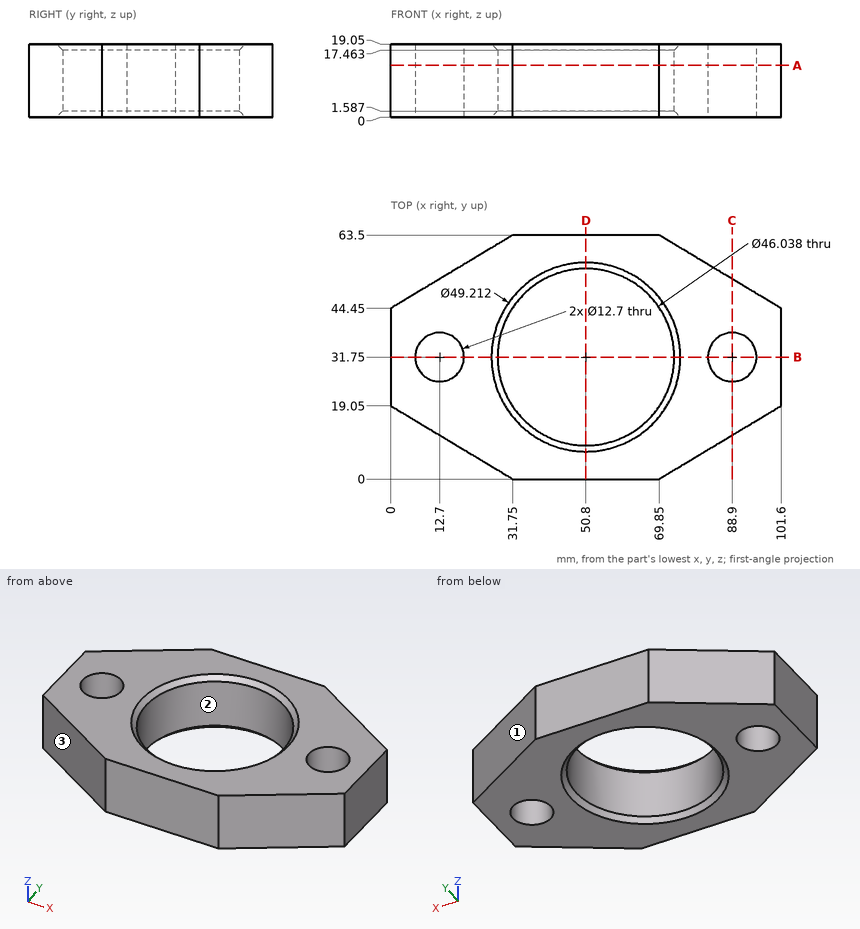
Job drawing, mm, ordinate dimensions from the low corner. One solid piece. Round coordinates to 2 decimals unless told otherwise and drop trailing zeros. Loops run counter-clockwise (first coordinate to the right, second up) from the corner with the lowest first, then second, coordinate; pieces in that order, holes last. Notation, with made-up numbers: (49, 82.5) -> (62, 82.5) arc R28 cw to (62, 117.5) -> close; hole circle Ø8 at (40.25, 30). An arc over 180 degrees is marked (long way). Use CSV: the item, a comma, the result in double quotes. Start each with the question number.
Q1. Mould opens along Y. For the marked faces 1, 2 and 3 say: +Y half, -Y half, draft (parallel to the pull), parting line (faces both ways), or undercut.
Q2. Drill centre lines: L1, parallel to X at y = 32, z = 6.5 (1 decimal); L2, parallel to Y at x = 40, z = 16.75; L3, parallel to Y at x = 88.9, z = 4.25. Where is each one in solid material? Low to high.
Q3. Saw through at B-B on y = 31.75. Give the cut face in (x, z).
Q4. Saw through at A-A on z = 13.5. Give the cut face in (x, y), and give its area (3 significant figures).
Q5. Saw through at C-C on x = 88.9. Give the cut face in (y, z), and give its area (3 significant figures).
Q6. Flat gauge pins, fed straight in: pin 1 Ø2 at (y, z) = (17.5, 9.5) entering from +X (1 decimal); pin 2 Ø8 at (x, z) = (20.5, 4.5) entering from -Y; pin 3 Ø7.5 at (x, y) = (12.7, 31.75) entering from +Z; pin 4 Ø2 at (x, z) = (72, 13.5) entering from +Y. Where does each tip first touch, or does it go through?
Q7. Saw through at D-D on x = 50.8. Give the cut face in (y, z).
Solutions:
1,face 1,"+Y half"
1,face 2,"undercut"
1,face 3,"-Y half"
2,L1,"x = 0 to 6.4, 19 to 27.8, 73.8 to 82.6, 95.2 to 101.6"
2,L2,"y = 0 to 11.42, 52.08 to 63.5"
2,L3,"y = 11.43 to 25.4, 38.1 to 52.07"
3,outline,"(0, 0) -> (6.35, 0) -> (6.35, 19.05) -> (0, 19.05) -> close; (19.05, 0) -> (26.19, 0) -> (27.78, 1.59) -> (27.78, 17.46) -> (26.19, 19.05) -> (19.05, 19.05) -> close; (73.82, 1.59) -> (75.41, 0) -> (82.55, 0) -> (82.55, 19.05) -> (75.41, 19.05) -> (73.82, 17.46) -> close; (95.25, 0) -> (101.6, 0) -> (101.6, 19.05) -> (95.25, 19.05) -> close"
4,outline,"(0, 19.05) -> (31.75, 0) -> (69.85, 0) -> (101.6, 19.05) -> (101.6, 44.45) -> (69.85, 63.5) -> (31.75, 63.5) -> (0, 44.45) -> close; hole circle Ø12.7 at (12.7, 31.75); hole circle Ø46.04 at (50.8, 31.75); hole circle Ø12.7 at (88.9, 31.75)"
4,area,"3,320 mm^2"
5,outline,"(11.43, 0) -> (25.4, 0) -> (25.4, 19.05) -> (11.43, 19.05) -> close; (38.1, 0) -> (52.07, 0) -> (52.07, 19.05) -> (38.1, 19.05) -> close"
5,area,"532 mm^2"
6,pin 1,"stops at x = 100.7"
6,pin 2,"stops at y = 4.35"
6,pin 3,"passes through"
6,pin 4,"stops at y = 62.81"
7,outline,"(0, 0) -> (7.14, 0) -> (8.73, 1.59) -> (8.73, 17.46) -> (7.14, 19.05) -> (0, 19.05) -> close; (54.77, 1.59) -> (56.36, 0) -> (63.5, 0) -> (63.5, 19.05) -> (56.36, 19.05) -> (54.77, 17.46) -> close"
